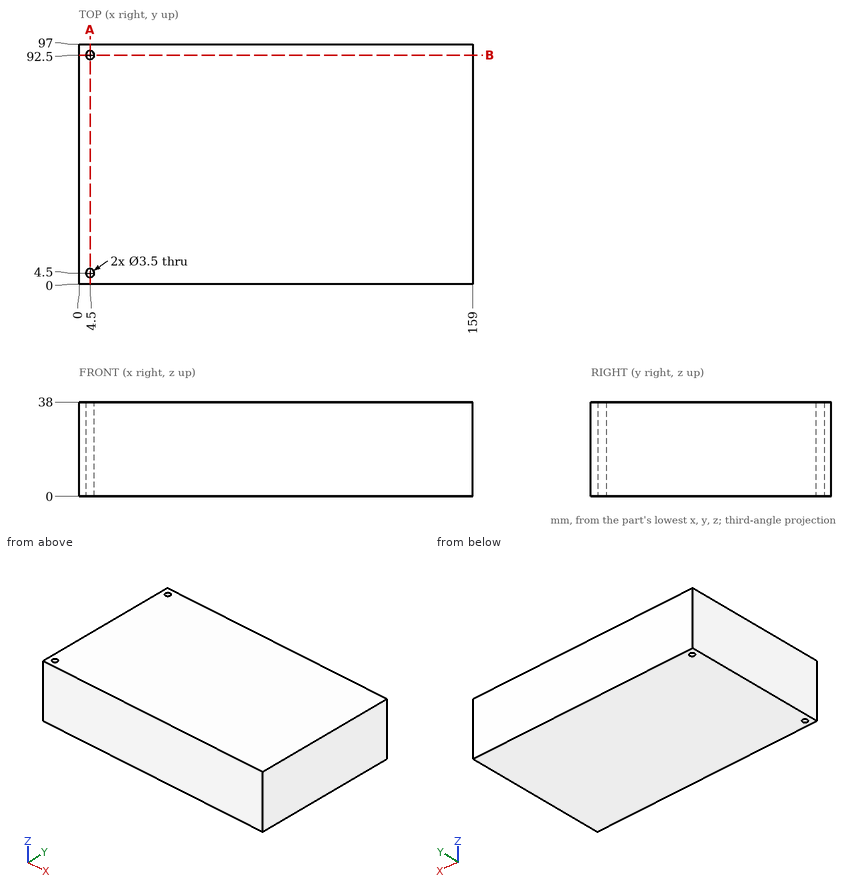
Can you work these out from the drawing? Everything is in mm from the part's minimum corner. Give positions to 0.01 mm unless a question says otherwise; leave off trailing zeros. Write each loop counter-clockwise with the first axis right and the second up, starting at its lowest first coordinate (ties: lowest second). Pieces come first, ordered by that corner, then holes. Notation, with made-up numbers: M 7,80.25 L 25,80.25 A11 ccw 25,94.25 Z; hole C 35.5,-4 d3. An arc over 180 degrees is marked long. Answer in a Markdown table with one row per item. Add a question column.
Item 1: Imagine slicing it at B-B, the plane y = 92.5. Write out the boundary of the cut face in (x, z), plus the area to 3 significant figures.
Item 2: Imagine slicing it at A-A, the plane x = 4.5. Write out the boundary of the cut face in (y, z).
Item 3: For pin 1 Ø2 at (x, y) = (4.5, 92.5) entering from +Z, with a flat end and sliding along its axis, tell me the tip position at first contact or that it passes through.
Item 4: Please list where these lines run through material, in increasing order: L1, parallel to Y at x = 4.5, z = 29; L2, parallel to X at y = 92.5, z = 22.5.
Evaluation:
| question | item | result |
|---|---|---|
| 1 | outline | M 0,0 L 2.75,0 L 2.75,38 L 0,38 Z; M 6.25,0 L 159,0 L 159,38 L 6.25,38 Z |
| 1 | area | 5,910 mm² |
| 2 | outline | M 0,0 L 2.75,0 L 2.75,38 L 0,38 Z; M 6.25,0 L 90.75,0 L 90.75,38 L 6.25,38 Z; M 94.25,0 L 97,0 L 97,38 L 94.25,38 Z |
| 3 | pin 1 | passes through |
| 4 | L1 | y = 0 to 2.75, 6.25 to 90.75, 94.25 to 97 |
| 4 | L2 | x = 0 to 2.75, 6.25 to 159 |
